For this review, take the finished solid that the model builds, in its own axes (mm). Coordinates: 2 decimals unless noted, no trailing zeros. Loops run counter-clockwise (first coordinate to the right, second up) from the corner with the lowest first, then second, coordinate; pieces in that order, holes last.
1. Take a section at D-D, the plane y = 190. State the section outline as (x, z) points, then the cut area to 3 significant figures.
2. To check wall thickness, follow probe 1 along Y at (x, z) = (0, 5); probe 2 along Y at (x, z) = (18, 5); probe 3 along X at (y, z) = (17, 5.75). State the ranges of each line that lie inside material, in increasing order.
3. Clearance check with flat-ended pins moving along their axes: P1, Ø4, axis at x = 16.5, z = 2.5, coming from the -Y side; P2, Ø6, axis at y = 183.5, z = 9.5, coming from the +X side. State where each tip first meets the part, or that it passes through.
4. Take a section at A-A, the plane x = 0. State the section outline as (y, z) points, then the cut area to 3 significant figures.
5. Mouldability with a two-part tool opening along Y and no side actions: class faces 1 (the face through (18, 330, 6)), 2 (the face through (-60, 138, 6)), 3 (the face through (78.476, 289.912, 5.916)) as pulls with the +Y half, pulls with the -Y half, needs draft (parallel to the pull), parting line crosses it, or undercut.
6. Take a section at C-C, the plane x = 17.5. State the section outline as (y, z) points.
7. Take a section at B-B, the plane z = 2.25. State the section outline as (x, y) points, then the cut area to 3 significant figures.
```python
from build123d import *

# Parameters (mm, degrees)
SKETCH_1_R      = 37.5
SKETCH_1_R_2    = 33
EXTRUDE_1_DEPTH = 12
FILLET_1_R      = 50


with BuildPart() as part:
    # 草图1 → 凸台-拉伸1 (new body)
    with BuildSketch(Plane.XY):
        with BuildLine():
            Line((-60, 0), (-60, 330))
            Line((-60, 330), (104, 330))
            Line((104, 330), (59.485849651, -7.837964739))
            ThreePointArc((59.485849651, -7.837964739), (-3.927405054, -59.871324435), (-60, 0))
        make_face()
        Circle(SKETCH_1_R, mode=Mode.SUBTRACT)
        with Locations((47, 280)):
            Circle(SKETCH_1_R_2, mode=Mode.SUBTRACT)
    extrude(amount=EXTRUDE_1_DEPTH)

    # 圆角1
    fillet_1_edges = [part.edges().sort_by_distance(p)[0] for p in [
        (-60, 330, 6),
        (104, 330, 6),
    ]]
    fillet(fillet_1_edges, radius=FILLET_1_R)


solid = part.part
```
Results list:
1. outline: (-60, 0) - (85.55, 0) - (85.55, 12) - (-60, 12) - close
1. area: 1,750 mm2
2. probe 1: y = -60 to -37.5, 37.5 to 330
2. probe 2: y = -57.24 to -32.9, 32.9 to 264.25, 295.75 to 330
2. probe 3: x = -60 to -33.43, 33.43 to 62.76
3. P1: stops at y = -58.22
3. P2: stops at x = 85.09
4. outline: (-60, 0) - (-37.5, 0) - (-37.5, 12) - (-60, 12) - close; (37.5, 0) - (330, 0) - (330, 12) - (37.5, 12) - close
4. area: 3,780 mm2
5. face 1: pulls with the +Y half
5. face 2: needs draft
5. face 3: undercut
6. outline: (-57.39, 0) - (-33.17, 0) - (-33.17, 12) - (-57.39, 12) - close; (33.17, 0) - (265.21, 0) - (265.21, 12) - (33.17, 12) - close; (294.79, 0) - (330, 0) - (330, 12) - (294.79, 12) - close
7. outline: (-60, 0) arc R60 ccw to (59.49, -7.84) - (96.55, 273.47) arc R50 ccw to (46.98, 330) - (-10, 330) arc R50 ccw to (-60, 280) - close; hole circle Ø75 at (0, 0); hole circle Ø66 at (47, 280)
7. area: 43,500 mm2
